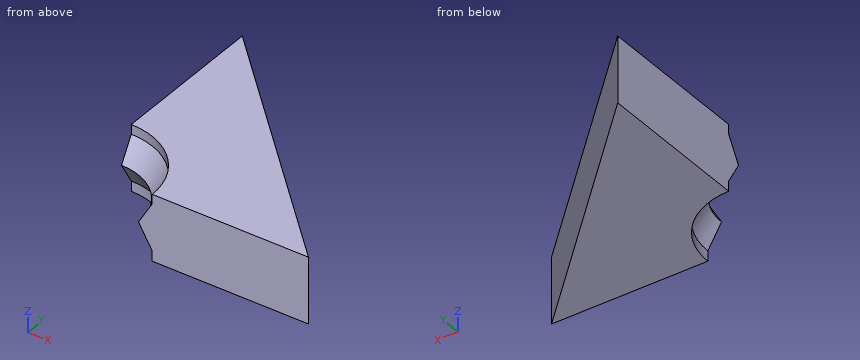
Autodesk Inventor part; units mm, degrees
ref_plane "YZ Plane" through (0, 0, 0) normal (1, 0, 0) x (0, 1, 0)
ref_plane "XZ Plane" through (0, 0, 0) normal (0, 1, 0) x (-1, 0, 0)
sketch "Sketch7" plane through (0, 0, 0) normal (0, 1, 0) x (-1, 0, 0)
  line L0 (0, 0) -> (0, 15.7673)
  line L1 (0, 0) -> (-13.3368, 0) construction
  line L2 (0, 15.7673) -> (-13.3368, 0) construction
  line L3 (0, 15.7673) -> (-18.6413, 0) construction
  line L4 (0, 15.7673) -> (-12.4569, -5.231) construction
  line L5 (0, 0) -> (0, -15.7673)
  line L6 (0, -15.7673) -> (-13.3368, 0) construction
  line L7 (0, -15.7673) -> (-18.6413, 0) construction
  line L8 (0, -15.7673) -> (-12.4569, 5.231) construction
  line L9 (-12.4569, 5.231) -> (-18.6413, 0) construction
  line L10 (-9.3537, 0) -> (-18.5948, -7.8164) construction
  line L11 (-9.3537, 0) -> (-18.0926, 7.3915) construction
  line L12 (0, -29.7093) -> (0, 66.7435)
  line L13 (-53.5, -5.9919) -> (-53.5, 6.008)
  line L14 (17.5786, 0) -> (-94.9714, 0)
  line L15 (-15.989, 2.2434) -> (-10.6846, -2.2434) construction
  line L16 (-10.6846, 2.2434) -> (-15.989, -2.2434) construction
  line L17 (-26.151, -15.9303) -> (-40.3783, -15.9303) construction
  line L18 (-40.3783, -15.9303) -> (-40.3783, -12.7539) construction
  line L19 (-40.3783, -12.7539) -> (-26.151, -12.7539) construction
  line L20 (-26.151, -12.7539) -> (-26.151, -15.9303) construction
  point P0 (-53.5, 0)
  dimension "Roller_Side_difference" = -0.0003
  dimension "d90" = 15.7673
  dimension "d201" = 53.5
  dimension "d343" = 99.548
  dimension "d344" = 99.549
  dimension "d367" = 8.1
sketch "Sketch44" plane through (0, 0, 0) normal (0, 1, 0) x (-1, 0, 0)
  line L0 (-18.7962, 0) -> (3.1509, -18.5634)
  line L1 (17.5786, 0) -> (-94.9714, 0)
  line L2 (-11.4508, 5.231) -> (-1, 5.231)
  line L3 (-14.3852, 5.231) -> (-53.5, 5.231)
  line L4 (0, 0) -> (0, 15.7673)
  line L5 (0, 0) -> (0, -15.8983)
  line L6 (-25.707, -7.6404) -> (3.3976, -7.6404)
  line L7 (-18.6413, 0) -> (0, -15.7673)
  point P0 (-3.6044, 0)
  point P1 (-9.6083, -7.6404)
  point P2 (0, -7.6404)
  dimension "d615" = 0.1
sketch "Sketch45" plane through (0, 0, 0) normal (0, 0, 1) x (1, 0, 0)
  line L0 (-12.5, 2.5) -> (12.5, 2.5)
  line L1 (12.5, 2.5) -> (12.5, -2.5)
  line L2 (12.5, -2.5) -> (-12.5, -2.5)
  line L3 (-12.5, -2.5) -> (-12.5, 2.5)
  line L4 (-12.5, 2.5) -> (12.5, -2.5) construction
  line L5 (12.5, 2.5) -> (-12.5, -2.5) construction
  point P0 (0, 0)
  dimension "d617" = 25
  dimension "d618" = 5
sketch "Sketch1" plane through (0, 0, 0) normal (0, 0, 1) x (1, 0, 0)
  circle A0 centre (0, 0) radius 13.3368 construction
  line L0 (0, 0) -> (13.3368, 0)
  line L1 (0, 0) -> (13.3368, 4.025)
  line L2 (13.3368, 0) -> (13.3368, 4.025)
  circle A1 centre (0, 0) radius 53.5
  point P0 (56.8, 0)
  dimension "d56" = 13.3368
  dimension "d57" = 4.025
  dimension "d400" = 53.5
  dimension "d495" = 2.5
  dimension "d496" = 8
  dimension "d531" = 5.5
  dimension "d532" = 5.5
  dimension "d533" = 5.5
  dimension "d537" = 24.5
  dimension "d538" = 3
  dimension "d543" = 5.5
  dimension "d549" = 3
  dimension "d550" = 3
  dimension "d567" = 5.5
  dimension "d568" = 5.5
sketch "Roller1" plane through (0, 0, 0) normal (0, 1, 0) x (-1, 0, 0)
  line L0 (0, 15.7673) -> (-12.4569, -5.231) construction
  line L1 (0, 15.7673) -> (-18.6413, 0) construction
  line L2 (-9.3537, 0) -> (-18.0926, 7.3915) construction
  line L3 (0, -15.7673) -> (-18.6413, 0) construction
  line L4 (-9.4248, -0.0708) -> (-12.4245, -5.1274)
  line L5 (-12.4245, -5.1274) -> (-18.5445, 0.0491)
  line L6 (-18.5445, 0.0491) -> (-14.0556, 3.846)
  line L7 (-14.0556, 3.846) -> (-9.4248, -0.0708)
  line L8 (-11.7456, 1.8921) -> (-15.4898, -2.5346)
  line L9 (-10.9821, 1.2463) -> (-14.7263, -3.1804)
  point P0 (0, 0)
  point P1 (-15.4845, -2.5391)
  dimension "d345" = 0.025
  dimension "d346" = 0.025
  dimension "d347" = 0.1
  dimension "d348" = 0.1
  dimension "d349" = 99.549
  dimension "d350" = 99.548
  dimension "d357" = 1
  dimension "d369" = 4.0148
sketch "Roller2" plane through (0, 0, 0) normal (0, 1, 0) x (-1, 0, 0)
  line L0 (0, -15.7673) -> (-12.4569, 5.231) construction
  line L1 (-9.3537, 0) -> (-18.5948, -7.8164) construction
  line L2 (0, -15.7673) -> (-18.6413, 0) construction
  line L3 (0, 15.7673) -> (-18.6413, 0) construction
  line L4 (-12.4245, 5.1274) -> (-9.4248, 0.0708)
  line L5 (-9.4248, 0.0708) -> (-14.0556, -3.846)
  line L6 (-14.0556, -3.846) -> (-18.5445, -0.0491)
  line L7 (-18.5445, -0.0491) -> (-12.4245, 5.1274)
  line L8 (-15.4845, 2.5391) -> (-11.7403, -1.8876)
  line L9 (-14.721, 3.1849) -> (-10.9767, -1.2418)
  point P0 (0, 0)
  dimension "d351" = 0.025
  dimension "d352" = 0.025
  dimension "d354" = 0.1
  dimension "d355" = 99.548
  dimension "d356" = 99.549
  dimension "d370" = 0.1
  dimension "d371" = 1
sketch "Sketch22" plane through (0, 0, 0) normal (0, 1, 0) x (-1, 0, 0)
  line L0 (-31.756, 8.0215) -> (-17.5287, 8.0215) construction
  line L1 (-17.5287, 8.0215) -> (-17.5287, 4.8451) construction
  line L2 (-17.5287, 4.8451) -> (-31.756, 4.8451) construction
  line L3 (-31.756, 4.8451) -> (-31.756, 8.0215) construction
  point P0 (0, 0)
  dimension "Roller_Side_difference" = -0.0003
sketch "Sketch2" plane through (0, 0, 0) normal (0, 1, 0) x (-1, 0, 0)
  line L0 (0, 0) -> (0, 13.3368) construction
  line L1 (0, 0) -> (-13.3368, 0)
  line L2 (0, 0) -> (0, -13.3368)
  line L3 (0, -13.3368) -> (-13.3368, 0) construction
  line L4 (0, 13.3368) -> (-13.3368, 0) construction
  line L5 (-78.8928, 52.9645) -> (0, 13.3368) construction
  line L6 (-34.8011, 15.91) -> (0, 13.3368) construction
  line L7 (-34.8011, 15.91) -> (0, -13.3368) construction
  line L8 (-48.3339, 16.9106) -> (0, -13.3368) construction
  point P0 (-17.4708, -4.134)
sketch "Sketch23" plane through (0, 0, 0) normal (0, 1, 0) x (-1, 0, 0)
  line L0 (0, -15.7673) -> (-12.4569, 5.231) construction
  line L1 (0, -15.7673) -> (-18.6413, 0) construction
  line L2 (0, 15.7673) -> (-12.4569, -5.231) construction
  line L3 (-12.4569, 5.231) -> (-18.6413, 0) construction
  line L4 (0, 15.7673) -> (-18.6413, 0) construction
  line L5 (-12.4569, 5.231) -> (-12.4569, -5.231) construction
  line L6 (17.5786, 0) -> (-94.9714, 0)
  line L7 (-11.4508, 3.731) -> (-9.2677, 0.051)
  line L8 (-9.2677, -0.051) -> (-11.4508, -3.731)
  line L9 (-14.3852, 3.731) -> (-18.7059, 0.0764)
  line L10 (-18.7059, -0.0764) -> (-14.3852, -3.731)
  arc A0 (-18.7059, 0.0764) -> (-18.7059, -0.0764) centre (-18.6413, 0) ccw
  arc A1 (-9.2677, -0.051) -> (-9.2677, 0.051) centre (-9.3537, 0) ccw
  line L11 (-11.4508, 3.731) -> (-11.4508, 5.231)
  line L12 (-11.4508, 5.231) -> (-1, 5.231)
  line L13 (-1, 5.231) -> (-1, -5.231)
  line L14 (-1, -5.231) -> (-11.4508, -5.231)
  line L15 (-11.4508, -5.231) -> (-11.4508, -3.731)
  line L16 (-14.3852, 3.731) -> (-14.3852, 5.231)
  line L17 (-14.3852, 5.231) -> (-53.5, 5.231)
  line L18 (-53.5, 5.231) -> (-53.5, -5.231)
  line L19 (-14.3852, -3.731) -> (-14.3852, -5.231)
  line L20 (-14.3852, -5.231) -> (-53.5, -5.231)
  line L21 (-12.4569, 5.231) -> (-12.4569, 5.231)
  line L22 (-12.4569, -5.231) -> (-12.4569, -5.231)
  line L23 (0, -29.7093) -> (0, 66.7435)
  line L24 (-18.7962, 0) -> (-53.5, 0)
  point P0 (0, 0)
  point P1 (-9.2374, 0)
  point P2 (-18.7413, 0)
  point P3 (-53.5, 0)
  dimension "d378" = 90
  dimension "d379" = 0.1
  dimension "d380" = 0.1
  dimension "d381" = 0.1
  dimension "d382" = 0.1
  dimension "d383" = 0.1
  dimension "d384" = 10.4619
  dimension "d385" = 0
  dimension "d386" = 0
  dimension "d391" = 1
  dimension "d392" = 53.5
  dimension "d393" = 1.5
  dimension "d394" = 1.5
  dimension "d395" = 1.5
  dimension "d396" = 1.5
sketch "Sketch46" plane through (0, 0, 0) normal (0, 1, 0) x (-1, 0, 0)
  line L0 (-11.4508, 3.731) -> (-9.2677, 0.051)
  line L1 (-9.2677, -0.051) -> (-11.4508, -3.731)
  arc A0 (-9.2677, -0.051) -> (-9.2677, 0.051) centre (-9.3537, 0) ccw
  line L2 (-11.4508, 3.731) -> (-11.4508, 5.231)
  line L3 (-11.4508, -5.231) -> (-11.4508, -3.731)
  line L4 (-11.5508, 5.231) -> (-11.5508, 3.7035)
  line L5 (-11.5508, 3.7035) -> (-9.3537, 0)
  line L6 (-9.3537, 0) -> (-11.5508, -3.7035)
  line L7 (-11.5508, -3.7035) -> (-11.5508, -5.3394)
  line L8 (-11.5508, 5.231) -> (-36.5508, 5.231)
  line L9 (-11.5508, -5.3394) -> (-36.5508, -5.3394)
  line L10 (-36.5508, -5.3394) -> (-36.5508, 5.231)
  line L11 (0, -29.7093) -> (0, 66.7435)
  point P0 (0, 0)
  dimension "d624" = 0.1
  dimension "d625" = 25
revolve "Revolution18" add sketch "Sketch46" angle 90 about axis through (0, 0, -10) along (0, 0, 1)
sketch "Sketch47" plane through (36.5508, 0, -5.3394) normal (0, 0, -1) x (-1, 0, 0)
  line L0 (36.5508, 36.5508) -> (0, 0)
  arc A0 (36.5508, 36.5508) -> (0, 0) centre (36.5508, 0) ccw
  point P0 (36.5508, 0)
extrude "Extrusion40" cut sketch "Sketch47" against normal through all
sketch "Sketch40" plane through (0, 0, -5.231) normal (0, 0, -1) x (-1, 0, 0)
  circle A0 centre (53.5, 0) radius 2.75
  circle A1 centre (0, 0) radius 53.5
  point P0 (53.4293, 2.7491)
  point P1 (53.4293, -2.7491)
  dimension "d585" = 8
  dimension "d587" = 1.75
  dimension "d589" = 3
  dimension "d592" = 2
  dimension "d593" = 12
  dimension "d594" = 12
  dimension "d611" = 360
equation "\"Roller_Side_difference\" = -0.001568deg"
equation "\"Cycloid_Top_Plate_Fasner_Inner\" = 61.25"
equation "\"Cycloid_Top_Plate_Fasner_Outer\" = 85.75"
equation "\"Roller_Hole_Radius\" = 1"
equation "\"Distance_To_Bearing\" = 20.65135"
equation "\"d514\" = 0.2"
properties part number "InnerRaceTool"
Model file for the job. Use its own axes, mm. Give positions to 0.01 mm unless a question says otherwise; leave off trailing zeros. Write each loop counter-clockwise with the first axis right and the second up, starting at its lowest first coordinate (ties: lowest second). Pieces come first, ordered by that corner, then holes. Notation, with made-up numbers: M 41,-28.5 L 97,-28.5 A27 ccw 97,4.5 Z; hole C 82,-36 d6. An arc over 180 degrees is marked long. Use a Markdown table: item, result.
1) Cut at A-A (y = 25). List the corners of the cut face in (x, z), and give its area (3 significant figures).
Responses:
| item | result |
|---|---|
| outline | M 0,-5.34 L 11.55,-5.34 L 11.55,5.23 L 0,5.23 Z |
| area | 122 mm2 |
2) Drill centre lines: line 1 (X direction, y = 6.5, z = 1.5); line 2 (X direction, y = 12, z = 2.5); line 3 (Y direction, x = 23.5, z = -3). Where is each one in solid material? Low to high. Write a range as from..to.
Responses:
| item | result |
|---|---|
| line 1 | x = 7.92..30.05 |
| line 2 | x = 0..24.55 |
| line 3 | y = 0..13.05 |
3) Cut at B-B (z = -4.5). List the corners of the cut face in (x, y).
Responses:
| item | result |
|---|---|
| outline | M 0,11.55 A11.55 cw 11.55,0 L 36.55,0 L 0,36.55 Z |
4) Pin check, flat tips, straight feed: pin 1 (2 mm diameter, centred on y = 7, z = 1.5, fed in from -X); pin 2 (3 mm diameter, centred on x = 32.5, z = 2, fed in from +Y); pin 3 (3 mm diameter, centred on x = 26, z = -4, fed in from -Y); pin 4 (5 mm diameter, centred on y = 19, z = 0, fed in from +X). Stop position of each tip, or through.
Responses:
| item | result |
|---|---|
| pin 1 | stops at x = 6.08 |
| pin 2 | stops at y = 5.55 |
| pin 3 | stops at y = 0 |
| pin 4 | stops at x = 20.05 |
